Can you work these out from the drawing? Everything is in mm from the part's minimum corner. Coordinates: 2 decimals unless noted, no trailing zeros. Order: outer loops, then holes, each group sorted by start corner. A loop starts at its lowest first (then second) coordinate and runs counter-clockwise, first axis right, second up. Notation, with made-up numbers: (35, 53) -> (91, 53) arc R21 ccw to (91, 80) -> close; hole circle Ø10 at (88.25, 33.25). An arc over 180 degrees is marked (long way). Use a Markdown table: item, result. Add a question column.
1) Will these pins go through, and if not, where does the flat tip stop? pin 1 Ø22 at (x, z) = (96.5, 14.5) entering from +Y; pin 2 Ø5 at (x, y) = (193.5, 6.5) entering from +Z; pin 3 Ø6 at (y, z) = (162.5, 11.5) entering from +X.
2) If we section it at B-B (y = 180.5): Write out the boundary of the cut face in (x, z), plus the area to 3 significant figures.
3) If we section it at A-A (z = 178.5): Write out the boundary of the cut face in (x, y).
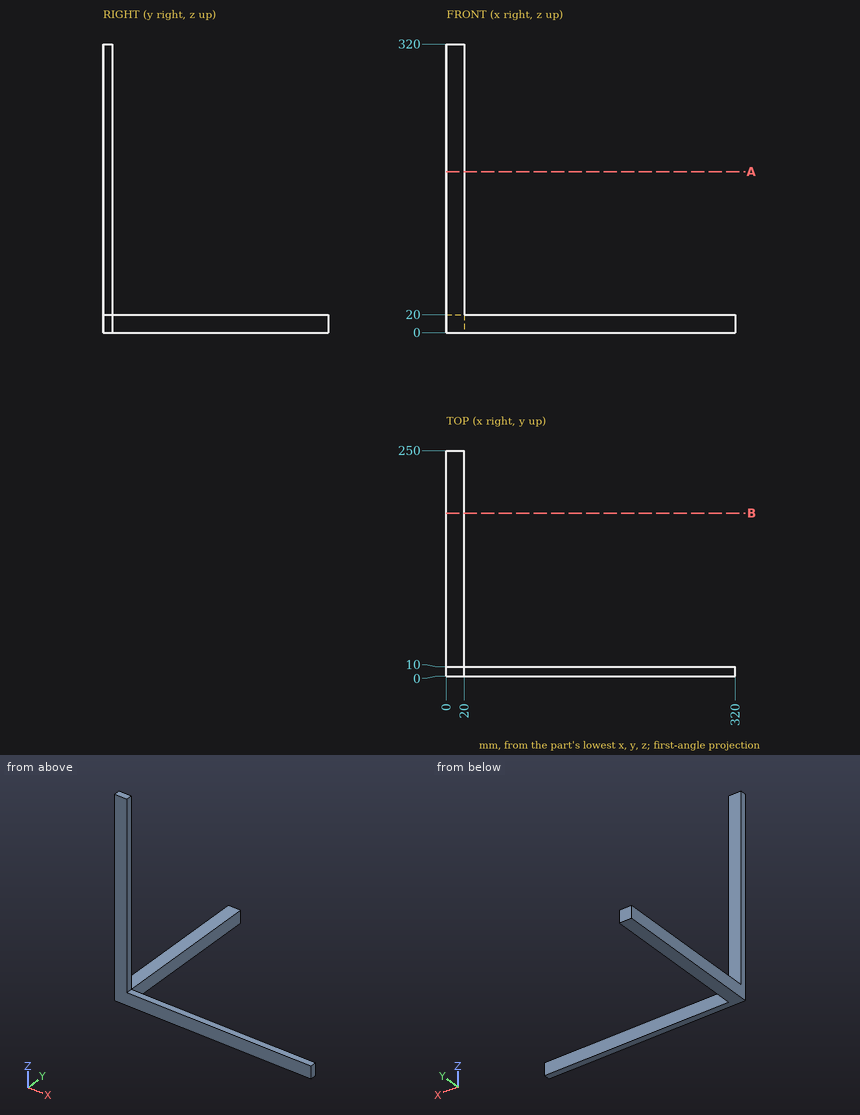
Answer sheet:
| question | item | result |
|---|---|---|
| 1 | pin 1 | y = 10 |
| 1 | pin 2 | z = 20 |
| 1 | pin 3 | x = 20 |
| 2 | outline | (0, 0) -> (20, 0) -> (20, 20) -> (0, 20) -> close |
| 2 | area | 400 mm2 |
| 3 | outline | (0, 0) -> (20, 0) -> (20, 10) -> (0, 10) -> close |
